Verification items for the finished model (mm, model axes). A direction names the side the tool comes from. Coordinates: 2 decimals unless noted, no trailing zeros. Write each loop counter-clockwise with the first axis right and the second up, starting at its lowest first coordinate (ties: lowest second). Pieces come first, ordered by that corner, then holes. Notation, with made-up numbers: (-27, 26) -> (-9, 26) arc R30 ccw to (-9, 63) -> close; hole circle Ø5 at (25, 29). An arc over 180 degrees is marked (long way). Answer in a Markdown table with one row per item.
```python
from build123d import *


with BuildPart() as part:
    # 草图1 → 旋转1 (revolve)
    with BuildSketch(Plane.XY, mode=Mode.PRIVATE) as revolve_1_sk:
        with BuildLine():
            Line((0, 76.25), (0, 71.75))
            Line((0, 71.75), (43.5, 71.75))
            Line((43.5, 71.75), (43.5, 76.25))
            Line((43.5, 76.25), (47.25, 76.25))
            Line((47.25, 76.25), (47.25, 88.915690404))
            ThreePointArc((47.25, 88.915690404), (34.625338065, 91.599539681), (21.7500009, 92.5))
            ThreePointArc((21.7500009, 92.5), (8.874662826, 91.599539806), (-3.75, 88.915690404))
            Line((-3.75, 88.915690404), (-3.75, 76.25))
            Line((-3.75, 76.25), (0, 76.25))
        make_face()
    revolve(revolve_1_sk.sketch.rotate(Axis((0, 0, 0), (1, 0, 0)), 90), axis=Axis((0, 0, 0), (1, 0, 0)))


solid = part.part
```
1. Tool access check on faces 1 (the flat face through (0, 50.5, -51.2)), 2 (the flat face through (43.5, 50.5, 51.2)), 3 (the cylindrical face through (22.054, -21.552, 68.437)). Record the directions out of +Z, -Z, +X, -X, +Y, -Y that give a thin tool (end or side, any length) a straight path to the whole face; none if there is none.
Geometry says:
| item | result |
|---|---|
| face 1 | -X |
| face 2 | +X |
| face 3 | +X, -X |
2. Thickness scan on line 1 (Y direction, x = 8.5, z = 0.5); line 2 (Y direction, x = 13, z = -18.5); line 3 (Z direction, x = 2, y = -11). Record the ranges inside material, lowest first. Write a range as from..to.
Geometry says:
| item | result |
|---|---|
| line 1 | -91.54..-71.75, 71.75..91.54 |
| line 2 | -90.21..-69.32, 69.32..90.21 |
| line 3 | -89.69..-70.9, 70.9..89.69 |
3. Depth check by flat-ended pin: P1, Ø2, axis at x = 13.5, y = 57, coming from the -Z side; P2, Ø3, axis at x = 25, z = 23, coming from the -Y side; P3, Ø1, axis at x = 10, y = 29, coming from the -Z side. Enter the tip coordinate at first touch or a pass-through.
Geometry says:
| item | result |
|---|---|
| P1 | z = -73.17 |
| P2 | y = -89.91 |
| P3 | z = -87.23 |
4. Mould release check, pull along Z, two halves, no side actions. Record for faces 4 (the cylindrical face through (45.4, -51.53, -56.2)), 5 (the flat face through (-3.75, -66, 39)): released by +Z, released by -Z, zero draft, split by the parting line, or undercut.
Geometry says:
| item | result |
|---|---|
| face 4 | undercut |
| face 5 | zero draft |
5. Section check A-A, the plane y = 0. Record the boundary of the cut face in (x, z), plus the area to 3 significant figures.
Geometry says:
| item | result |
|---|---|
| outline | (-3.75, -88.92) arc R92.5 ccw to (47.25, -88.92) -> (47.25, -76.25) -> (43.5, -76.25) -> (43.5, -71.75) -> (0, -71.75) -> (0, -76.25) -> (-3.75, -76.25) -> close; (-3.75, 76.25) -> (0, 76.25) -> (0, 71.75) -> (43.5, 71.75) -> (43.5, 76.25) -> (47.25, 76.25) -> (47.25, 88.92) arc R92.5 ccw to (-3.75, 88.92) -> close |
| area | 1,930 mm^2 |
6. Section check C-C, the plane x = 31. Record the boundary of the cut face in (y, z), plus the area to 3 significant figures.
Geometry says:
| item | result |
|---|---|
| outline | circle Ø184.07 at (0, 0); hole circle Ø143.5 at (0, 0) |
| area | 10,400 mm^2 |
7. Section check D-D, the plane z = 74. Record the boundary of the cut face in (x, y), plus the area to 3 significant figures.
Geometry says:
| item | result |
|---|---|
| outline | (-3.75, -49.3) arc R55.5 ccw to (47.25, -49.3) -> (47.25, -18.39) -> (43.5, -18.39) -> (43.5, 18.39) -> (47.25, 18.39) -> (47.25, 49.3) arc R55.5 ccw to (-3.75, 49.3) -> (-3.75, 18.39) -> (0, 18.39) -> (0, -18.39) -> (-3.75, -18.39) -> close |
| area | 5,180 mm^2 |
